```python
from build123d import *

# Parameters (mm, degrees)
SKETCH1_W           = 23
SKETCH1_H           = 23
BOSS_EXTRUDE1_DEPTH = 10
SKETCH2_R           = 2.5
SKETCH2_R_2         = 6
BOSS_EXTRUDE2_DEPTH = 5


with BuildPart() as part:
    # Sketch1 → Boss-Extrude1 (new body)
    with BuildSketch(Plane.XY):
        Rectangle(SKETCH1_W, SKETCH1_H)
        Polygon((-2.5, 10), (-10, 10), (-10, 2.5), (-6, 2.5), (-6, -2.5), (-10, -2.5), (-10, -10), (-2.5, -10), (-2.5, -6), (2.5, -6), (2.5, -10), (10, -10), (10, -2.5), (6, -2.5), (6, 2.5), (10, 2.5), (10, 10), (2.5, 10), (2.5, 6), (-2.5, 6), align=None, mode=Mode.SUBTRACT)
    extrude(amount=BOSS_EXTRUDE1_DEPTH)

    # Sketch2 → Boss-Extrude2 (add)
    with BuildSketch(Plane(origin=(0, 11.5, 0), x_dir=(1, 0, 0), z_dir=(0, 1, 0))):
        with BuildLine():
            Line((-12, -20.506265624), (-12, 10.506265624))
            ThreePointArc((-12, 10.506265624), (0, 22.506265624), (12, 10.506265624))
            Line((12, 10.506265624), (12, -20.506265624))
            ThreePointArc((12, -20.506265624), (0, -32.506265624), (-12, -20.506265624))
        make_face()
        with Locations(Location((0, 10, 0), (0, 0, 270))):
            Circle(SKETCH2_R, mode=Mode.SUBTRACT)
        with Locations(Location((0, -20, 0), (0, 0, 90))):
            Circle(SKETCH2_R, mode=Mode.SUBTRACT)
        with Locations(Location((0, -5, 0), (0, 0, 56.442690238))):
            Circle(SKETCH2_R_2, mode=Mode.SUBTRACT)
    extrude(amount=BOSS_EXTRUDE2_DEPTH)


solid = part.part
```
Design review of the part built by this model. Coordinates are the model's own, in mm. A direction names the side the tool comes from. Give positions to 0.01 mm unless a question says otherwise; leave off trailing zeros. Order: outer loops, then holes, each group sorted by start corner. A loop starts at its lowest first (then second) coordinate and runs counter-clockwise, first axis right, second up. Notation, with made-up numbers: (57, 89) -> (108, 89) arc R25 ccw to (108, 118) -> close; hole circle Ø7 at (2, 15). An arc over 180 degrees is marked (long way). Write item = value, one per line. Start each with the question number.
(1) We need section C-C on x = -0.75. Write out the cut boundary in (y, z).
(2) We need section D-D on x = 8.25. Write out the cut boundary in (y, z), plus the area to 3 significant figures.
(3) To check wall thickness, follow line 1 along X through (y, z) = (9.5, 2.5); line 2 along Y through (x, z) = (-4.5, 5.5); line 3 along X through (y, z) = (13.7, 20). State the ranges of each line that lie inside material, in increasing order.
(4) Mouldability with a two-part tool opening along Y and no side actions: class faces 4 (the face through (-6, 10, 5)), 5 (the face through (12, 14, 5)), 6 (the face through (0, 11.5, 5)) as +Y half, -Y half, draft (parallel to the pull), parting line (faces both ways), or undercut.
(5) For faces 1 (the face through (11.5, 0, 5)), 2 (the face through (2.5, -8, 5)), 3 (the face through (-11.5, 0, 5)), list the 3-axis set-ups (+Z, -Z, +X, -X, +Y, -Y) from which the entire face can be reached by the end or side of a thin tool; tool diameter is ignored.
(6) We need section A-A on y = 0.75. Write out the cut boundary in (x, z), plus the area to 3 significant figures.
(7) For pin 1 (8 mm diameter, centred on x = 7, z = 16.5, fed in from -Y); pin 2 (9.5 mm diameter, centred on x = 0, z = 5, fed in from +Y); pin 3 (11 mm diameter, centred on y = 1, z = 3.5, fed in from -X), all flat-tipped, find the tip position at first contact; note any pin that passes through.
Numbers:
q1.outline = (-11.5, 0) -> (-6, 0) -> (-6, 10) -> (-11.5, 10) -> close; (6, 0) -> (11.5, 0) -> (11.5, 10) -> (6, 10) -> close; (11.5, -22.48) -> (16.5, -22.48) -> (16.5, -12.38) -> (11.5, -12.38) -> close; (11.5, -7.62) -> (16.5, -7.62) -> (16.5, -0.95) -> (11.5, -0.95) -> close; (11.5, 10.95) -> (16.5, 10.95) -> (16.5, 17.62) -> (11.5, 17.62) -> close; (11.5, 22.38) -> (16.5, 22.38) -> (16.5, 32.48) -> (11.5, 32.48) -> close
q2.outline = (-11.5, 0) -> (-10, 0) -> (-10, 10) -> (-11.5, 10) -> close; (-2.5, 0) -> (2.5, 0) -> (2.5, 10) -> (-2.5, 10) -> close; (10, 0) -> (11.5, 0) -> (11.5, -19.22) -> (16.5, -19.22) -> (16.5, 29.22) -> (11.5, 29.22) -> (11.5, 10) -> (10, 10) -> close
q2.area = 322 mm^2
q3.line_1 = -11.5 to -10, -2.5 to 2.5, 10 to 11.5
q3.line_2 = -11.5 to -10, 10 to 11.5
q3.line_3 = -12 to -2.5, 2.5 to 12
q4.face_4 = undercut
q4.face_5 = draft
q4.face_6 = +Y half
q5.face_1 = +Z, -Z, +X, -Y
q5.face_2 = +Z, -Z
q5.face_3 = +Z, -Z, -X, -Y
q6.outline = (-11.5, 0) -> (-6, 0) -> (-6, 10) -> (-11.5, 10) -> close; (6, 0) -> (11.5, 0) -> (11.5, 10) -> (6, 10) -> close
q6.area = 110 mm^2
q7.pin_1 = 11.5
q7.pin_2 = 11.5
q7.pin_3 = -11.5
